The model under review builds one solid part; all positions refer to its coordinate system, in mm. Face numbers are marked on the shaded views. A direction names the side the tool comes from. Coordinates: 2 decimals unless noted, no trailing zeros. Loops run counter-clockwise (first coordinate to the right, second up) from the corner with the lowest first, then second, coordinate; pieces in that order, holes last. Notation, with made-up numbers: (-3.75, -12) - (33.25, -12) arc R24 cw to (33.25, -1) - close; hole circle Ø4 at (84, 85). An arc over 180 degrees is marked (long way). One line per item, written item: value. Start each with the question number.
1. We need section C-C, the plane y = 0. Give the boundary of the cut face in (x, z), then the cut area to 3 significant figures.
2. We need section A-A, the plane x = 0. Give the boundary of the cut face in (y, z).
3. Insertion check: P1, Ø1, axis at y = -2, z = -2, coming from the +X side; P2, Ø1.5, axis at y = 6, z = -1, coming from the -X side; P3, Ø1, axis at y = -11.5, z = 2.5, coming from the -X side. Each pin has a flat end and moves straight along its axis. Give the tip position at first contact, or say it passes through.
4. For the marked faces 5, 6, 7 and 8, list the 3-axis set-ups (+Z, -Z, +X, -X, +Y, -Y) from which the entire face can be reached by the end or side of a thin tool; tool diameter is ignored.
5. To check wall thickness, follow line 1 (X direction, y = 0.5, z = 0); line 2 (Y direction, x = 2, z = -0.5); line 3 (Y direction, x = 1, z = 1.5). State the ranges of each line that lie inside material, in increasing order.
6. Mouldability with a two-part tool opening along Y and no side actions: class the marked faces 1, 2, 3 and 4 as +Y half, -Y half, draft (parallel to the pull), parting line (faces both ways), or undercut.
7. We need section D-D, the plane x = -13.5. Give the boundary of the cut face in (y, z).
from build123d import *

# Parameters (mm, degrees)
BOSS_EXTRUDE1_DEPTH      = 5
BOSS_EXTRUDE1_DEPTH_BACK = 5
SKETCH1_R                = 10
SKETCH1_R_2              = 6


with BuildPart() as part:
    # Sketch1 → Boss-Extrude1 (new, two sides: drawn at the far end of the back side and taken through both)
    # profile 1 of 6: a face of its own
    with BuildSketch(Plane.XY.offset(-BOSS_EXTRUDE1_DEPTH_BACK)):
        Circle(SKETCH1_R)
        Circle(SKETCH1_R_2, mode=Mode.SUBTRACT)
    # profile 2 of 6: a face of its own
    with BuildSketch(Plane.XY.offset(-BOSS_EXTRUDE1_DEPTH_BACK)):
        with BuildLine():
            Line((-1, -17.5), (1, -17.5))
            Line((1, -17.5), (2.215917914, -16.523588481))
            Line((2.215917914, -16.523588481), (3.826834324, -9.238795325))
            ThreePointArc((3.826834324, -9.238795325), (1.95090322, -9.807852804), (0, -10))
            ThreePointArc((0, -10), (-1.95090322, -9.807852804), (-3.826834324, -9.238795325))
            Line((-3.826834324, -9.238795325), (-2.215917914, -16.523588481))
            Line((-2.215917914, -16.523588481), (-1, -17.5))
        make_face()
    # profile 3 of 6: a face of its own
    with BuildSketch(Plane.XY.offset(-BOSS_EXTRUDE1_DEPTH_BACK)):
        with BuildLine():
            Line((-15.030110204, -7.21353282), (-7.604059656, -6.494480483))
            ThreePointArc((-7.604059656, -6.494480483), (-8.724960071, -4.886212415), (-9.510565163, -3.090169944))
            ThreePointArc((-9.510565163, -3.090169944), (-9.93068457, -1.175373975), (-9.969173337, 0.784590957))
            Line((-9.969173337, 0.784590957), (-16.399622791, -2.998606477))
            Line((-16.399622791, -2.998606477), (-16.95250603, -4.456740885))
            Line((-16.95250603, -4.456740885), (-16.334472041, -6.358853918))
            Line((-16.334472041, -6.358853918), (-15.030110204, -7.21353282))
        make_face()
    # profile 4 of 6: a face of its own
    with BuildSketch(Plane.XY.offset(-BOSS_EXTRUDE1_DEPTH_BACK)):
        with BuildLine():
            Line((-11.505036874, 12.065380019), (-8.526401644, 5.224985647))
            ThreePointArc((-8.526401644, 5.224985647), (-7.343225094, 6.788007455), (-5.877852523, 8.090169944))
            ThreePointArc((-5.877852523, 8.090169944), (-4.186597375, 9.081431738), (-2.334453639, 9.723699204))
            Line((-2.334453639, 9.723699204), (-7.919606374, 14.670347759))
            Line((-7.919606374, 14.670347759), (-9.477224921, 14.745582654))
            Line((-9.477224921, 14.745582654), (-11.095258909, 13.570012149))
            Line((-11.095258909, 13.570012149), (-11.505036874, 12.065380019))
        make_face()
    # profile 5 of 6: a face of its own
    with BuildSketch(Plane.XY.offset(-BOSS_EXTRUDE1_DEPTH_BACK)):
        with BuildLine():
            ThreePointArc((5.877852523, 8.090169944), (7.343225094, 6.788007455), (8.526401644, 5.224985647))
            Line((8.526401644, 5.224985647), (11.505036874, 12.065380019))
            Line((11.505036874, 12.065380019), (11.095258909, 13.570012149))
            Line((11.095258909, 13.570012149), (9.477224921, 14.745582654))
            Line((9.477224921, 14.745582654), (7.919606374, 14.670347759))
            Line((7.919606374, 14.670347759), (2.334453639, 9.723699204))
            ThreePointArc((2.334453639, 9.723699204), (4.186597375, 9.081431738), (5.877852523, 8.090169944))
        make_face()
    # profile 6 of 6: a face of its own
    with BuildSketch(Plane.XY.offset(-BOSS_EXTRUDE1_DEPTH_BACK)):
        with BuildLine():
            ThreePointArc((9.510565163, -3.090169944), (8.724960071, -4.886212415), (7.604059656, -6.494480483))
            Line((7.604059656, -6.494480483), (15.030110204, -7.21353282))
            Line((15.030110204, -7.21353282), (16.334472041, -6.358853918))
            Line((16.334472041, -6.358853918), (16.95250603, -4.456740885))
            Line((16.95250603, -4.456740885), (16.399622791, -2.998606477))
            Line((16.399622791, -2.998606477), (9.969173337, 0.784590957))
            ThreePointArc((9.969173337, 0.784590957), (9.992290362, 0.392598158), (10, 0))
            ThreePointArc((10, 0), (9.876883406, -1.56434465), (9.510565163, -3.090169944))
        make_face()
    extrude(amount=BOSS_EXTRUDE1_DEPTH + BOSS_EXTRUDE1_DEPTH_BACK)


solid = part.part
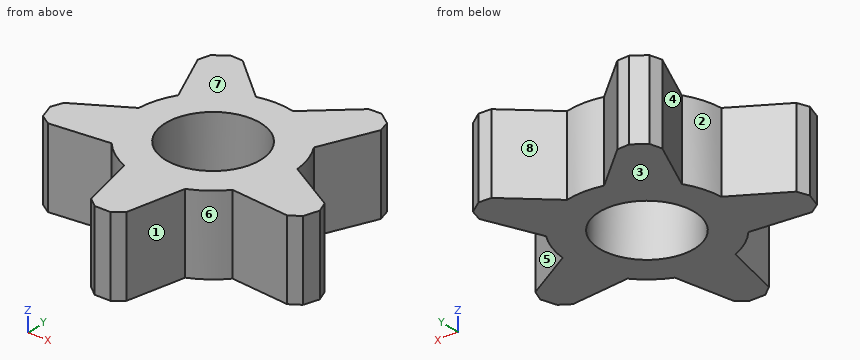
Findings below:
1. outline: (-11.3, -5) - (-6, -5) - (-6, 5) - (-11.3, 5) - close; (6, -5) - (11.3, -5) - (11.3, 5) - (6, 5) - close
1. area: 106 mm2
2. outline: (-17.5, -5) - (-6, -5) - (-6, 5) - (-17.5, 5) - close; (6, -5) - (10, -5) - (10, 5) - (6, 5) - close
3. P1: x = 15.55
3. P2: x = -9.19
3. P3: x = -3.44
4. face 5: +Z, -Z, +X
4. face 6: +Z, -Z, -Y
4. face 7: +Z, +X, -X, +Y, -Y
4. face 8: +Z, -Z, +Y
5. line 1: -10.45 to -5.98, 5.98 to 10.45
5. line 2: -16.7 to -5.66, 5.66 to 9.8
5. line 3: -17.5 to -5.92, 5.92 to 9.95
6. face 1: -Y half
6. face 2: undercut
6. face 3: draft
6. face 4: undercut
7. outline: (-7.07, -5) - (-1.29, -5) - (-1.29, 5) - (-7.07, 5) - close
